Model file for the job. Use its own axes, mm. Face numbers are marked on the shaded views. A direction names the side the tool comes from. Round coordinates to 2 decimals unless told otherwise and drop trailing zeros. Loops run counter-clockwise (first coordinate to the right, second up) from the corner with the lowest first, then second, coordinate; pieces in that order, holes last. Notation, with made-up numbers: (64, -28) -> (106, -28) arc R14 cw to (106, -1) -> close; hole circle Ø4 at (-28.5, 34.5). An arc over 180 degrees is marked (long way). Use a Markdown table: item, result. Add a question column.
Solid Edge part; units mm, degrees
sketch "Sketch1" plane through (0, 0, 0) normal (0, -1, 0) x (1, 0, 0)
  circle A0 centre (27.94, 50.285) radius 1.5
  line L0 (30.94, 53.285) -> (-30.94, 53.285)
  line L1 (-30.94, 53.285) -> (-30.94, -53.285)
  line L2 (-30.94, -53.285) -> (30.94, -53.285)
  line L3 (30.94, -53.285) -> (30.94, 53.285)
  circle A1 centre (-27.94, -50.285) radius 1.5
  circle A2 centre (-27.94, 50.285) radius 1.5
  circle A3 centre (27.94, -50.285) radius 1.5
extrude "Protrusion1" add sketch "Sketch1" against normal blind 1.4
sketch "Sketch2" plane through (0, 0, 0) normal (0, -1, 0) x (1, 0, 0)
  line L0 (30.44, 47.285) -> (-30.44, 47.285)
  line L1 (-30.44, 47.285) -> (-30.44, -47.285)
  line L2 (-30.44, -47.285) -> (30.44, -47.285)
  line L3 (30.44, -47.285) -> (30.44, 47.285)
  line L4 (27.84, 44.685) -> (-27.84, 44.685)
  line L5 (-27.84, 44.685) -> (-27.84, -38.835)
  line L6 (-27.84, -38.835) -> (27.84, -38.835)
  line L7 (27.84, -38.835) -> (27.84, 44.685)
extrude "ExtrudedProtrusion_2" add sketch "Sketch2" along normal blind 4
sketch "Sketch3" plane through (0, 0, 0) normal (0, -1, 0) x (1, 0, 0)
  line L0 (27.84, 44.685) -> (-27.84, 44.685)
  line L1 (-27.84, 44.685) -> (-27.84, -38.835)
  line L2 (-27.84, -38.835) -> (27.84, -38.835)
  line L3 (27.84, -38.835) -> (27.84, 44.685)
extrude "ExtrudedProtrusion_3" add sketch "Sketch3" along normal blind 2.229
sketch "Sketch4" plane through (0, 0, 0) normal (0, -1, 0) x (1, 0, 0)
  line L0 (12.7, 52.555) -> (-12.7, 52.555)
  line L1 (-12.7, 52.555) -> (-12.7, 50.015)
  line L2 (-12.7, 50.015) -> (12.7, 50.015)
  line L3 (12.7, 50.015) -> (12.7, 52.555)
extrude "ExtrudedProtrusion_4" add sketch "Sketch4" against normal blind 2.4
sketch "Sketch5" plane through (0, 1.4, 0) normal (0, 1, 0) x (-1, 0, 0)
  line L0 (16.9211, -14.7927) -> (16.9211, -7.556)
  line L1 (16.9211, -7.556) -> (-16.9211, -7.556)
  line L2 (-16.9211, -7.556) -> (-16.9211, -14.7927)
  line L3 (-16.9211, -14.7927) -> (16.9211, -14.7927)
extrude "ExtrudedProtrusion_5" add sketch "Sketch5" along normal blind 2
sketch "Sketch6" plane through (0, 0, 0) normal (0, -1, 0) x (1, 0, 0)
  line L0 (27.84, 44.685) -> (-27.84, 44.685)
  line L1 (-27.84, 44.685) -> (-27.84, -38.835)
  line L2 (-27.84, -38.835) -> (27.84, -38.835)
  line L3 (27.84, -38.835) -> (27.84, 44.685)
extrude "ExtrudedProtrusion_6" add sketch "Sketch6" along normal blind 3.9
properties material "Polycarbonate"
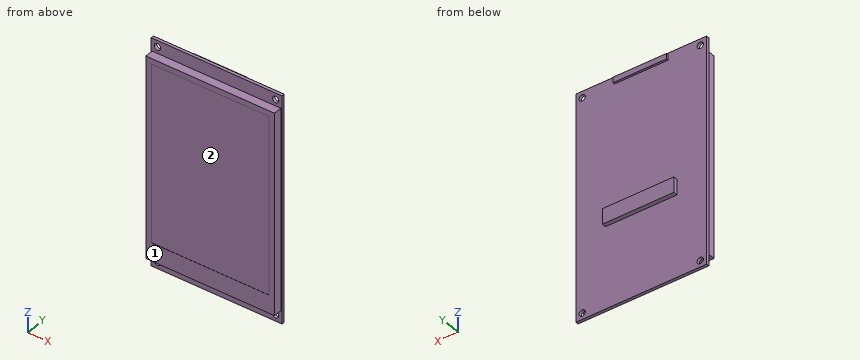
1) Cut at C-C on y = -1.5. Write the cut outline in (x, z) (3 decimals), and give its area (3 significant figures).
2) Pin check, flat tips, straight feed: pin 1 Ø1.1 at (x, y) = (4, 2) entering from -Z; pin 2 Ø3.5 at (x, z) = (27.94, 50.285) entering from +Y; pin 3 Ø1 at (x, z) = (-1.5, 3.5) entering from -Y. Stop position of each tip, or through.
3) Cut at B-B on z = -21. Write the cut outline in (x, y).
4) Cut at D-D on x = 3. Write the cut outline in (y, z) (3 decimals), and give its area (3 significant figures).
5) Wall check: probe 1 along Z at (x, y) = (-27.94, 0.75) (3 decimals); probe 2 along Z at (x, y) = (-0.5, 1.5) (3 decimals); probe 3 along Y at (x, z) = (24, 33.5). Give the ranges that are in metal, low to high. Write a range as from..to.
6) Cut at A-A on x = 21.5. Write the cut outline in (y, z) (3 decimals).
7) Tool access for the marked faces 1 and 2: list every direction of +Z, -Z, +X, -X, +Y, -Y with a clear straight run to the whole face (end or side of a thin tool).
Established:
| question | item | result |
|---|---|---|
| 1 | outline | (-30.44, -47.285) -> (30.44, -47.285) -> (30.44, 47.285) -> (-30.44, 47.285) -> close |
| 1 | area | 5,760 mm^2 |
| 2 | pin 1 | stops at z = -14.79 |
| 2 | pin 2 | stops at y = 1.4 |
| 2 | pin 3 | stops at y = -3.9 |
| 3 | outline | (-30.94, 0) -> (-30.44, 0) -> (-30.44, -4) -> (-27.84, -4) -> (-27.84, -3.9) -> (27.84, -3.9) -> (27.84, -4) -> (30.44, -4) -> (30.44, 0) -> (30.94, 0) -> (30.94, 1.4) -> (-30.94, 1.4) -> close |
| 4 | outline | (-4, -47.285) -> (0, -47.285) -> (0, -53.285) -> (1.4, -53.285) -> (1.4, -14.793) -> (3.4, -14.793) -> (3.4, -7.556) -> (1.4, -7.556) -> (1.4, 50.015) -> (2.4, 50.015) -> (2.4, 52.555) -> (1.4, 52.555) -> (1.4, 53.285) -> (0, 53.285) -> (0, 47.285) -> (-4, 47.285) -> (-4, 44.685) -> (-3.9, 44.685) -> (-3.9, -38.835) -> (-4, -38.835) -> close |
| 4 | area | 536 mm^2 |
| 5 | probe 1 | z = -53.285..-51.785, -48.785..48.785, 51.785..53.285 |
| 5 | probe 2 | z = -14.793..-7.556, 50.015..52.555 |
| 5 | probe 3 | y = -3.9..1.4 |
| 6 | outline | (-4, -47.285) -> (0, -47.285) -> (0, -53.285) -> (1.4, -53.285) -> (1.4, 53.285) -> (0, 53.285) -> (0, 47.285) -> (-4, 47.285) -> (-4, 44.685) -> (-3.9, 44.685) -> (-3.9, -38.835) -> (-4, -38.835) -> close |
| 7 | face 1 | +Z, -Z, +X, -X, -Y |
| 7 | face 2 | -Y |
